Geometry check sheet. Reference: the model listing, model coordinates, mm. Face numbers are marked on the shaded views. A direction names the side the tool comes from. Give positions to 0.01 mm unless a question says otherwise; leave off trailing zeros. Order: outer loops, then holes, each group sorted by start corner. A loop starts at its lowest first (then second) coordinate and runs counter-clockwise, first axis right, second up.
from build123d import *

# Parameters (mm, degrees)
SKETCH1_W           = 40
SKETCH1_H           = 43
SKETCH1_R           = 2
BOSS_EXTRUDE1_DEPTH = 4
SKETCH4_W           = 40
SKETCH4_H           = 3
BOSS_EXTRUDE2_DEPTH = 40
SKETCH5_R           = 1.5
SKETCH5_R_2         = 10
CUT_EXTRUDE1_DEPTH  = 24
BOSS_EXTRUDE3_DEPTH = 2
BOSS_EXTRUDE4_DEPTH = 2


with BuildPart() as part:
    # Sketch1 → Boss-Extrude1 (new body)
    with BuildSketch(Plane(origin=(0, 0, 0), x_dir=(1, 0, 0), z_dir=(0, 1, 0))):
        Rectangle(SKETCH1_W, SKETCH1_H)
        with Locations(Location((-14.715053003, 12, 0), (0, 0, 270))):
            Circle(SKETCH1_R, mode=Mode.SUBTRACT)
        with Locations(Location((15.284946997, 12, 0), (0, 0, 270))):
            Circle(SKETCH1_R, mode=Mode.SUBTRACT)
        with Locations(Location((-14.715053003, -12, 0), (0, 0, 270))):
            Circle(SKETCH1_R, mode=Mode.SUBTRACT)
        with Locations(Location((15.284946997, -12, 0), (0, 0, 270))):
            Circle(SKETCH1_R, mode=Mode.SUBTRACT)
    extrude(amount=-BOSS_EXTRUDE1_DEPTH)

    # Sketch4 → Boss-Extrude2 (add)
    with BuildSketch(Plane(origin=(0, 0, 0), x_dir=(1, 0, 0), z_dir=(0, 1, 0))):
        with Locations((0, 20)):
            Rectangle(SKETCH4_W, SKETCH4_H)
    extrude(amount=BOSS_EXTRUDE2_DEPTH)

    # Sketch5 → Cut-Extrude1 (cut)
    with BuildSketch(Plane.XY.offset(-18.5)):
        with Locations((8.491960292, 37.449274423)):
            Circle(SKETCH5_R)
        with Locations((-13.72832995, 28.379616129)):
            Circle(SKETCH5_R)
        with Locations((5.236369657, 13.671109447)):
            Circle(SKETCH5_R)
        with Locations((0, 26.5)):
            Circle(SKETCH5_R_2)
    extrude(amount=-CUT_EXTRUDE1_DEPTH, mode=Mode.SUBTRACT)

    # Sketch6 → Boss-Extrude3 (add)
    with BuildSketch(Plane(origin=(20, 0, 0), x_dir=(0, 0, -1), z_dir=(1, 0, 0))):
        Polygon((18.5, 15), (3.5, 0), (18.5, 0), align=None)
    extrude(amount=-BOSS_EXTRUDE3_DEPTH)

    # Sketch7 → Boss-Extrude4 (add)
    with BuildSketch(Plane.ZY.offset(20)):
        Polygon((-18.5, 15), (-3.5, 0), (-18.5, 0), align=None)
    extrude(amount=-BOSS_EXTRUDE4_DEPTH)


solid = part.part
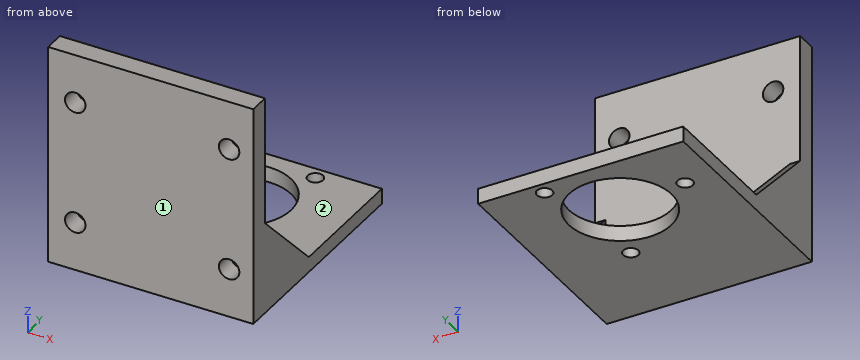
Item 1: Sectioned sample at B-B (x = -6). Enter the section's corners in (y, z), and give its area (3 significant figures).
Reported:
outline: (-4, -21.5) - (18.5, -21.5) - (18.5, -18.5) - (0, -18.5) - (0, 21.5) - (-4, 21.5) - close; (34.5, -21.5) - (40, -21.5) - (40, -18.5) - (34.5, -18.5) - close
area: 244 mm2
Item 2: Set-up check for the marked faces 1 and 2: record each of +Z, -Z, +X, -X, +Y, -Y from which the full face is reachable in a straight line by a thin tool's end or side.
Reported:
face 1: +Z, -Z, +X, -X, -Y
face 2: +Z, +Y
Item 3: Sectioned sample at A-A (z = 12). Enter the section's corners in (x, y), and give its area (3 significant figures).
Reported:
outline: (-20, -4) - (-16.72, -4) - (-16.72, 0) - (-20, 0) - close; (-12.72, -4) - (13.28, -4) - (13.28, 0) - (-12.72, 0) - close; (17.28, -4) - (20, -4) - (20, 0) - (17.28, 0) - close
area: 128 mm2
Item 4: Scan lines: L1, parallel to X at y = -1, z = -12; L2, parallel to X at y = 7, z = -13.5; L3, parallel to Y at x = -14, z = 3. Record each from-to range of solid material in increasing order.
Reported:
L1: x = -20 to -16.72, -12.72 to 13.28, 17.28 to 20
L2: x = -20 to -18, 18 to 20
L3: y = -4 to 0
Item 5: Sectioned sample at C-C (y = 7). Enter the section's corners in (x, z).
Reported:
outline: (-20, -21.5) - (20, -21.5) - (20, -10.5) - (18, -10.5) - (18, -18.5) - (-18, -18.5) - (-18, -10.5) - (-20, -10.5) - close
Item 6: Gauge pin test, flat ends, axial feed: pin 1 (20 mm diameter, centred on x = 7, z = 3.5, fed in from +Y); pin 2 (1.5 mm diameter, centred on x = -4.5, y = 8.5, fed in from +Z); pin 3 (2.5 mm diameter, centred on x = -13.73, y = 28.38, fed in from +Z). Record the tip position at first contact, or that the pin passes through.
Reported:
pin 1: stops at y = 0
pin 2: stops at z = -18.5
pin 3: passes through
Item 7: Sectioned sample at D-D (y = 27.5). Enter the section's corners in (x, z), and give its area (3 significant figures).
Reported:
outline: (-20, -21.5) - (-14.94, -21.5) - (-14.94, -18.5) - (-20, -18.5) - close; (-12.51, -21.5) - (-9.95, -21.5) - (-9.95, -18.5) - (-12.51, -18.5) - close; (9.95, -21.5) - (20, -21.5) - (20, -18.5) - (9.95, -18.5) - close
area: 53.0 mm2
